Can you work these out from the model? Positions are in its coordinate system, mm. A direction names the side the tool comes from. Coordinates: 2 decimals unless noted, no trailing zeros. Order: outer loops, then holes, each group sorted by start corner. A loop starts at its lowest first (then second) coordinate and runs counter-clockwise, first axis right, second up. Notation, with made-up numbers: M 17.5,41 L 43.5,41 A16 cw 43.5,59 Z; hole C -11.5,12 d6. An arc over 180 degrees is marked long. Answer as a JSON object with one key per item and string values.
Autodesk Inventor part; units mm, degrees
ref_plane "YZ Plane" through (0, 0, 0) normal (1, 0, 0) x (0, 1, 0)
ref_plane "XZ Plane" through (0, 0, 0) normal (0, 1, 0) x (-1, 0, 0)
ref_plane "XY Plane" through (0, 0, 0) normal (0, 0, 1) x (1, 0, 0)
sketch "Sketch1" plane through (0, 0, 0) normal (1, 0, 0) x (0, 1, 0)
  line L0 (10.6126, 22.7394) -> (-14.3874, 22.7394)
  line L1 (-14.3874, 22.7394) -> (-14.3874, -12.2606)
  line L2 (-14.3874, -12.2606) -> (10.6126, -12.2606)
  line L3 (10.6126, -12.2606) -> (10.6126, 22.7394)
  line L4 (5.7696, 24.7394) -> (3.7696, 24.7394)
  line L5 (3.7696, 24.7394) -> (3.7696, 22.7394)
  line L6 (3.7696, 22.7394) -> (5.7696, 22.7394)
  line L7 (5.7696, 22.7394) -> (5.7696, 24.7394)
  line L8 (-6.5839, 24.7394) -> (-8.5839, 24.7394)
  line L9 (-8.5839, 24.7394) -> (-8.5839, 22.7394)
  line L10 (-8.5839, 22.7394) -> (-6.5839, 22.7394)
  line L11 (-6.5839, 22.7394) -> (-6.5839, 24.7394)
  line L12 (3.7696, 22.7394) -> (-6.5839, 22.7394)
  point P0 (0, 0)
  dimension "d0" = 25
  dimension "d1" = 35
  dimension "d2" = 2
  dimension "d3" = 2
  dimension "d4" = 2
  dimension "d5" = 2
extrude "Extrusion1" add sketch "Sketch1" along normal blind 2
properties part number "sidestandforservoclamp"
Item 1: If we mould it in two halves opening along Y, with no side actions, what happens to faces 1 (the flat face through (1, -8, 24.739)), 2 (the flat face through (1, -14.387, 5)), 3 (the flat face through (1, 3.77, 24))? For each: pulls with the +Y half, pulls with the -Y half, needs draft (parallel to the pull), parting line crosses it, or undercut.
Answers follow:
{"face 1": "needs draft", "face 2": "pulls with the -Y half", "face 3": "undercut"}
Item 2: Which directions (+Z, -Z, +X, -X, +Y, -Y) give clear straight access to the entire face, cutting with the end or side of a thin tool? Please do faces 4 (the flat face through (2, -2, 6)), 5 (the flat face through (1, -11, 22.739)), 6 (the flat face through (1, 5.77, 24)), 7 (the flat face through (1, -1, 22.739)), 8 (the flat face through (1, -2, -12.261)).
Answers follow:
{"face 4": "+Z, -Z, +X, +Y, -Y", "face 5": "+Z, +X, -X, -Y", "face 6": "+Z, +X, -X, +Y", "face 7": "+Z, +X, -X", "face 8": "-Z, +X, -X, +Y, -Y"}
Item 3: I'm going to push a flat-ended pin straight in: pin 1 (1 mm diameter, centred on x = 1, y = 0, fed in from +Z). Where does the tip first touch, or does it pass through?
Answers follow:
{"pin 1": "stops at z = 22.74"}
Item 4: I want a section at A-A, the plane x = 0.4. Write out the boundary of the cut face in (y, z).
Answers follow:
{"outline": "M -14.39,-12.26 L 10.61,-12.26 L 10.61,22.74 L 5.77,22.74 L 5.77,24.74 L 3.77,24.74 L 3.77,22.74 L -6.58,22.74 L -6.58,24.74 L -8.58,24.74 L -8.58,22.74 L -14.39,22.74 Z"}
Item 5: Please list where this line runs through material, in increasing order: line 1 (Z direction, x = 1.6, y = -4.25).
Answers follow:
{"line 1": "z = -12.26 to 22.74"}
Item 6: I want a section at B-B, the plane y = 8.75. Write out the boundary of the cut face in (x, z), plus the area to 3 significant figures.
Answers follow:
{"outline": "M 0,-12.26 L 2,-12.26 L 2,22.74 L 0,22.74 Z", "area": "70.0 mm^2"}
